For this review, take the finished solid that the model builds, in its own axes (mm). A direction names the side the tool comes from. Coordinates: 2 decimals unless noted, no trailing zeros. Order: outer loops, then holes, each group sorted by start corner. A loop starts at its lowest first (then second) coordinate and runs counter-clockwise, first axis right, second up. Notation, with made-up numbers: (67, -10) -> (75, -10) arc R19 cw to (75, 14) -> close; hole circle Ø8 at (-19, 80.25). An arc over 180 degrees is marked (long way). Answer as a JSON object with one key per item and string values. Group by question number.
1) Add section C-C, the plane y = 1.7. Write out the cut boundary in (x, z) (3 decimals).
2) Add section D-D, the plane x = 58.5. Write out the cut boundary in (y, z) (3 decimals).
3) Add section A-A, the plane x = -67.2. Write out the cut boundary in (y, z) (3 decimals), then the cut area to 3 significant figures.
4) Draft analysis for pull direction X (two halves, no side actions). For faces 3 (the cylindrical face through (-76.77, 1.61, -26)), 4 (the flat face through (-73.39, 2, 0)), 5 (the cylindrical face through (76.7, 1.61, 26.07)), 6 (the flat face through (0, 2, -17.465)), state which applies: +X half, -X half, draft (parallel to the pull), parting line (faces both ways), or undercut.
5) Machinability: for faces 1 (the flat face through (-1, 0, -13)), 2 (the flat face through (10, 2, -20)), which of the approach directions +Z, -Z, +X, -X, +Y, -Y give a long, thin tool a straight path to every point of the face, cutting with its end or side? Answer none if there is none.
6) Wall thickness on L1, parallel to Z at x = -67.2, y = 1.8; L2, parallel to X at y = 0.9, z = -20.5; L3, parallel to X at y = 3.05, z = 4.5: over which ranges is each line inside the solid? List them lowest first.
7) Add section B-B, the plane z = 20.5. Write out the cut boundary in (x, y) (3 decimals).
from build123d import *

# Parameters (mm, degrees)
SKETCH1_W           = 156.4
SKETCH1_H           = 55
BOSS_EXTRUDE1_DEPTH = 3.175
SKETCH2_R           = 1.6
CUT_EXTRUDE1_DEPTH  = 83.955232656
SKETCH5_W           = 146.78
SKETCH5_H           = 24.86
CUT_EXTRUDE4_DEPTH  = 3.175
SKETCH6_W           = 20
SKETCH6_H           = 5
CUT_EXTRUDE5_DEPTH  = 83.955232656
FILLET1_R           = 5


with BuildPart() as part:
    # Sketch1 → Boss-Extrude1 (new body)
    with BuildSketch(Plane(origin=(0, 0, 0), x_dir=(1, 0, 0), z_dir=(0, 1, 0))):
        Rectangle(SKETCH1_W, SKETCH1_H)
    extrude(amount=BOSS_EXTRUDE1_DEPTH)

    # Sketch2 → Cut-Extrude1 (cut, through all)
    with BuildSketch(Plane.XZ):
        with Locations(Location((67.2, 20.5, 0), (0, 0, 270))):
            Circle(SKETCH2_R)
        with Locations(Location((67.2, -20.5, 0), (0, 0, 270))):
            Circle(SKETCH2_R)
        with Locations(Location((-67.2, -20.5, 0), (0, 0, 270))):
            Circle(SKETCH2_R)
        with Locations(Location((-67.2, 20.5, 0), (0, 0, 270))):
            Circle(SKETCH2_R)
    extrude(amount=-CUT_EXTRUDE1_DEPTH, mode=Mode.SUBTRACT)

    # Sketch5 → Cut-Extrude4 (cut)
    with BuildSketch(Plane.XZ):
        Rectangle(SKETCH5_W, SKETCH5_H)
    extrude(amount=-CUT_EXTRUDE4_DEPTH, mode=Mode.SUBTRACT)

    # Sketch6 → Cut-Extrude5 (cut, through all)
    with BuildSketch(Plane(origin=(0, 0, 0), x_dir=(-1, 0, 0), z_dir=(0, -1, 0))):
        with Locations((0, -19.965)):
            Rectangle(SKETCH6_W, SKETCH6_H)
        with Locations((0, 19.965)):
            Rectangle(SKETCH6_W, SKETCH6_H)
    extrude(amount=-CUT_EXTRUDE5_DEPTH, mode=Mode.SUBTRACT)

    # Fillet1
    fillet1_edges = [part.edges().sort_by_distance(p)[0] for p in [
        (78.2, 1.5875, 27.5),
        (-78.2, 1.5875, 27.5),
        (-78.2, 1.5875, -27.5),
        (78.2, 1.5875, -27.5),
    ]]
    fillet(fillet1_edges, radius=FILLET1_R)


solid = part.part
Output values:
{
 "1": {"outline": "(-78.2, -22.5) arc R5 ccw to (-73.2, -27.5) -> (73.2, -27.5) arc R5 ccw to (78.2, -22.5) -> (78.2, 22.5) arc R5 ccw to (73.2, 27.5) -> (-73.2, 27.5) arc R5 ccw to (-78.2, 22.5) -> close; hole (-73.39, -12.43) -> (73.39, -12.43) -> (73.39, 12.43) -> (-73.39, 12.43) -> close; hole circle Ø3.2 at (-67.2, -20.5); hole circle Ø3.2 at (-67.2, 20.5); hole (-10, -22.465) -> (10, -22.465) -> (10, -17.465) -> (-10, -17.465) -> close; hole (-10, 17.465) -> (10, 17.465) -> (10, 22.465) -> (-10, 22.465) -> close; hole circle Ø3.2 at (67.2, -20.5); hole circle Ø3.2 at (67.2, 20.5)"},
 "2": {"outline": "(0, -27.5) -> (3.175, -27.5) -> (3.175, -12.43) -> (0, -12.43) -> close; (0, 12.43) -> (3.175, 12.43) -> (3.175, 27.5) -> (0, 27.5) -> close"},
 "3": {"outline": "(0, -27.5) -> (3.175, -27.5) -> (3.175, -22.1) -> (0, -22.1) -> close; (0, -18.9) -> (3.175, -18.9) -> (3.175, -12.43) -> (0, -12.43) -> close; (0, 12.43) -> (3.175, 12.43) -> (3.175, 18.9) -> (0, 18.9) -> close; (0, 22.1) -> (3.175, 22.1) -> (3.175, 27.5) -> (0, 27.5) -> close", "area": "75.4 mm²"},
 "4": {"face 3": "-X half", "face 4": "undercut", "face 5": "+X half", "face 6": "undercut"},
 "5": {"face 1": "+Z, -Z, +X, -X, -Y", "face 2": "+Y, -Y"},
 "6": {"L1": "z = -27.5 to -22.1, -18.9 to -12.43, 12.43 to 18.9, 22.1 to 27.5", "L2": "x = -78.2 to -68.8, -65.6 to -10, 10 to 65.6, 68.8 to 78.2", "L3": "x = -78.2 to -73.39, 73.39 to 78.2"},
 "7": {"outline": "(-78.2, 0) -> (-68.8, 0) -> (-68.8, 3.175) -> (-78.2, 3.175) -> close; (-65.6, 0) -> (-10, 0) -> (-10, 3.175) -> (-65.6, 3.175) -> close; (10, 0) -> (65.6, 0) -> (65.6, 3.175) -> (10, 3.175) -> close; (68.8, 0) -> (78.2, 0) -> (78.2, 3.175) -> (68.8, 3.175) -> close"}
}
